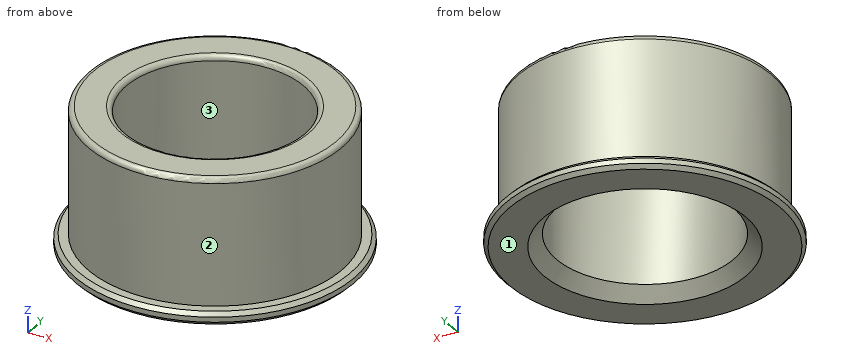
```python
from build123d import *

# Parameters (mm, degrees)
SKETCH2_R           = 10
SKETCH2_R_2         = 7
BOSS_EXTRUDE1_DEPTH = 10
BOSS_EXTRUDE2_START = -1
SKETCH2_3_R         = 11
SKETCH2_3_R_2       = 10
SKETCH2_3_R_3       = 7
BOSS_EXTRUDE2_DEPTH = 1
CHAMFER1_SIZE       = 0.3
CHAMFER2_SIZE       = 0.3
CHAMFER3_SIZE       = 1
FILLET1_R           = 0.4


with BuildPart() as part:
    # Sketch2 → Boss-Extrude1 (new body)
    with BuildSketch(Plane.XY):
        Circle(SKETCH2_R)
        Circle(SKETCH2_R_2, mode=Mode.SUBTRACT)
    extrude(amount=BOSS_EXTRUDE1_DEPTH)

    # Sketch2_3 → Boss-Extrude2 (add)
    # profile 1 of 2: a face of its own
    with BuildSketch(Plane.XY.offset(BOSS_EXTRUDE2_START)):
        Circle(SKETCH2_3_R)
        Circle(SKETCH2_3_R_2, mode=Mode.SUBTRACT)
    # profile 2 of 2: a face of its own
    with BuildSketch(Plane.XY.offset(BOSS_EXTRUDE2_START)):
        Circle(SKETCH2_3_R_2)
        Circle(SKETCH2_3_R_3, mode=Mode.SUBTRACT)
    extrude(amount=BOSS_EXTRUDE2_DEPTH)

    # Chamfer1
    chamfer1_edges = [part.edges().sort_by_distance(p)[0] for p in [
        (-11, 0, 0),
    ]]
    chamfer(chamfer1_edges, length=CHAMFER1_SIZE)

    # Chamfer2
    chamfer2_edges = [part.edges().sort_by_distance(p)[0] for p in [
        (-11, 0, -1),
    ]]
    chamfer(chamfer2_edges, length=CHAMFER2_SIZE)

    # Chamfer3
    chamfer3_edges = [part.edges().sort_by_distance(p)[0] for p in [
        (-7, 0, -1),
    ]]
    chamfer(chamfer3_edges, length=CHAMFER3_SIZE)

    # Fillet1
    fillet1_edges = [part.edges().sort_by_distance(p)[0] for p in [
        (-10, 0, 10),
        (-7, 0, 10),
    ]]
    fillet(fillet1_edges, radius=FILLET1_R)


solid = part.part
```
Check sheet for the modelled part. Datum: model origin and axes. Units: mm. Face numbers are marked on the shaded views. Give positions to 0.01 mm unless a question says otherwise; leave off trailing zeros. Order: outer loops, then holes, each group sorted by start corner. A loop starts at its lowest first (then second) coordinate and runs counter-clockwise, first axis right, second up. Notation, with made-up numbers: M -18,-10 L 29,-10 A9 cw 29,4 Z; hole C 46.5,70.5 d8. An arc over 180 degrees is marked long. Answer in a Markdown table with one row per item.
1) Release check for a two-part mould opening along Y. For the marked faces 1, 2 and 3 record: +Y half, -Y half, draft (parallel to the pull), parting line (faces both ways), or undercut.
Filled sheet:
| item | result |
|---|---|
| face 1 | draft |
| face 2 | parting line |
| face 3 | undercut |
2) Cross-section at A-A, the plane x = 0. Enter the section's corners in (y, z).
Filled sheet:
| item | result |
|---|---|
| outline | M -11,-0.7 L -10.7,-1 L -8,-1 L -7,0 L -7,9.6 A0.4 ccw -7.4,10 L -9.6,10 A0.4 ccw -10,9.6 L -10,0 L -10.7,0 L -11,-0.3 Z; M 7,0 L 8,-1 L 10.7,-1 L 11,-0.7 L 11,-0.3 L 10.7,0 L 10,0 L 10,9.6 A0.4 ccw 9.6,10 L 7.4,10 A0.4 ccw 7,9.6 Z |
3) Cross-section at C-C, the plane z = 7.5. Enter the section's corners in (x, y).
Filled sheet:
| item | result |
|---|---|
| outline | C 0,0 d20; hole C 0,0 d14 |
4) Gauge pin test, flat ends, axial feed: P1, Ø10.5, axis at x = 5, y = 1.5, coming from the +Z side; P2, Ø2, axis at x = 4, z = 5.5, coming from the +Y side; P3, Ø6, axis at x = 5.5, z = 6.5, coming from the +Y side; P4, Ø1.5, axis at x = 0, z = 1.5, coming from the -Y side. Record the tip position at first contact, or that the pin passes through.
Filled sheet:
| item | result |
|---|---|
| P1 | stops at z = 10 |
| P2 | stops at y = 9.54 |
| P3 | stops at y = 9.68 |
| P4 | stops at y = -10 |
5) Thickness scan on L1, parallel to Y at x = 0, z = 3.5; L2, parallel to X at y = 3.5, z = 7. Record the ranges inside material, lowest first. Write a range as [from, to].
Filled sheet:
| item | result |
|---|---|
| L1 | y = [-10, -7], [7, 10] |
| L2 | x = [-9.37, -6.06], [6.06, 9.37] |
